from build123d import *

# Parameters (mm, degrees)
F0_W     = 450
F0_H     = 450
F1_DEPTH = 950
F2_W     = 46.0927397013
F2_H     = 50
F2_W_2   = 333.9072602987
F2_H_2   = 425
F3_DEPTH = 450.001
F4_W     = 398.5071629286
F4_H     = 74.7186541557
F4_W_2   = 401.3135582209
F4_H_2   = 287.5961661339
F5_DEPTH = 413.0608200261
F6_W     = 380
F6_H     = 425
F7_DEPTH = 450.001
F8_W     = 380
F8_H     = 305.6115476475
F8_H_2   = 50
F9_DEPTH = 126.5918704384


with BuildPart() as f1:
    # F0 (on Top) → F1 (new body)
    with BuildSketch(Plane.XY):
        Rectangle(F0_W, F0_H)
    extrude(amount=F1_DEPTH)

    # F2 (on face) → F3 (cut, through all)
    with BuildSketch(Plane.YZ.offset(225)):
        with Locations((201.9536301494, 450)):
            Rectangle(F2_W, F2_H)
        Polygon((-225, 950), (-225, 475), (143.9072602987, 475), (190, 950), align=None)
        Polygon((225, 950), (178.9072602987, 475), (225, 475), align=None)
        with Locations((-23.0463698506, 212.5)):
            Rectangle(F2_W_2, F2_H_2)
        with Locations((201.9536301494, 212.5)):
            Rectangle(F2_W, F2_H_2)
    extrude(amount=-F3_DEPTH, mode=Mode.SUBTRACT)

    # F4 (on face) → F5 (cut, through all)
    with BuildSketch(Plane(origin=(0, 96.9020668341, -9.4031194592), x_dir=(1, 0, 0), z_dir=(0, -0.9953248675, 0.0965836843))):
        with Locations((-1.3172850013, 884.6258819103)):
            Rectangle(F4_W, F4_H)
        with Locations((0.0859126449, 651.3064205647)):
            Rectangle(F4_W_2, F4_H_2)
    extrude(amount=F5_DEPTH, mode=Mode.SUBTRACT)

    # F6 (on face) → F7 (cut, through all)
    with BuildSketch(Plane.XZ.offset(225)):
        with Locations((0, 212.5)):
            Rectangle(F6_W, F6_H)
    extrude(amount=-F7_DEPTH, mode=Mode.SUBTRACT)

    # F8 (on face) → F9 (cut, through all)
    with BuildSketch(Plane(origin=(0, 96.9020668341, -9.4031194592), x_dir=(1, 0, 0), z_dir=(0, -0.9953248675, 0.0965836843))):
        with Locations((0, 639.4841792974)):
            Rectangle(F8_W, F8_H)
        with Locations((0, 867.2899531212)):
            Rectangle(F8_W, F8_H_2)
    extrude(amount=-F9_DEPTH, mode=Mode.SUBTRACT)


solid = f1.part
CAD build for the part. Positions are in the model's coordinates, mm. A direction names the side the tool comes from. Coordinates: 2 decimals unless noted, no trailing zeros. Write each loop counter-clockwise with the first axis right and the second up, starting at its lowest first coordinate (ties: lowest second). Pieces come first, ordered by that corner, then holes. Notation, with made-up numbers: (53.25, 33.25) - (61.25, 33.25) arc R25 cw to (61.25, 63.25) - close; hole circle Ø2 at (59, 48). An arc over 180 degrees is marked (long way). Use a Markdown table: item, result. Add a question column.
Item 1: Band-saw the part on C-C, the plane z = 513. Give the cut face in (x, y), and give its area (3 significant figures).
Item 2: Flat gauge pins, fed straight in: pin 1 (12 mm diameter, centred on x = 21, y = -131.5, fed in from -Z); pin 2 (5 mm diameter, centred on x = 17.5, y = 31.5, fed in from +Z); pin 3 (17.5 mm diameter, centred on x = 210.5, z = 171.5, fed in from +Y). Where does each tip first touch, or does it go through?
Item 3: Mould opens along X. For faces 5 (the face through (16, -225, 430)), 6 (the face through (-190, 176, 623)), 7 (the face through (225, 16, 438)) say: pulls with the +X half, pulls with the -X half, needs draft (parallel to the pull), parting line crosses it, or undercut.
Item 4: Band-saw the part on D-D, the plane y = -31.5. Give the cut face in (x, z), and give its area (3 significant figures).
Item 5: Band-saw the part on A-A, the plane x = 31. Give the cut face in (y, z), and give its area (3 significant figures).
Item 6: Drill centre lines: L1, parallel to X at y = -195, z = 171.5; L2, parallel to Y at x = 34, z = 460; L3, parallel to Z at x = 179, y = -56. Where is each one in solid material? Low to high. Write a range as from..to.
Item 7: Band-saw the part on B-B, the plane z = 180. Give the cut face in (x, y).
Item 8: 3-axis set-ups, long thin cutter, end or side, ignore diameter. For faces 1 (the face through (3, -43, 475)), 2 (the face through (190, -208, 210)), 3 (the face through (-207, -190, 210)), 4 (the face through (-2.66, 195.35, 827.29)): which of +Z, -Z, +X, -X, +Y, -Y reach the whole face in a straight line?
Numbers:
| question | item | result |
|---|---|---|
| 1 | outline | (-225, 147.59) - (-190, 147.59) - (-190, 182.59) - (-225, 182.59) - close; (190, 147.59) - (225, 147.59) - (225, 182.59) - (190, 182.59) - close |
| 1 | area | 2,450 mm2 |
| 2 | pin 1 | z = 425 |
| 2 | pin 2 | z = 475 |
| 2 | pin 3 | y = 178.91 |
| 3 | face 5 | needs draft |
| 3 | face 6 | undercut |
| 3 | face 7 | pulls with the +X half |
| 4 | outline | (-225, 425) - (225, 425) - (225, 475) - (-225, 475) - close |
| 4 | area | 22,500 mm2 |
| 5 | outline | (-225, 425) - (178.91, 425) - (178.91, 471.6) - (143.91, 475) - (-225, 475) - close; (173.42, 779.18) - (208.1, 775.82) - (212.93, 825.58) - (178.25, 828.95) - close; (183.08, 878.72) - (217.76, 875.35) - (225, 950) - (190, 950) - close |
| 5 | area | 24,400 mm2 |
| 6 | L1 | -225..-190, 190..225 |
| 6 | L2 | -225..178.91 |
| 6 | L3 | 425..475 |
| 7 | outline | (-225, -225) - (-190, -225) - (-190, -190) - (-225, -190) - close; (-225, 143.91) - (-190, 143.91) - (-190, 178.91) - (-225, 178.91) - close; (190, -225) - (225, -225) - (225, -190) - (190, -190) - close; (190, 143.91) - (225, 143.91) - (225, 178.91) - (190, 178.91) - close |
| 8 | face 1 | +Z, +X, -X, -Y |
| 8 | face 2 | -Z, +Y, -Y |
| 8 | face 3 | -Z, +X, -X |
| 8 | face 4 | +Y |
